Could you check a few things on this model? Use its own coordinates, in mm. Coordinates: 2 decimals unless noted, no trailing zeros. One line per item, written item: value.
Autodesk Inventor part; units mm, degrees
ref_plane "YZ Plane" through (0, 0, 0) normal (1, 0, 0) x (0, 1, 0)
ref_plane "XZ Plane" through (0, 0, 0) normal (0, 1, 0) x (-1, 0, 0)
ref_plane "XY Plane" through (0, 0, 0) normal (0, 0, 1) x (1, 0, 0)
sketch "Sketch1" plane through (0, 0, 0) normal (0, 1, 0) x (-1, 0, 0)
  line L0 (-0.4496, -84) -> (-0.4496, 0)
  line L1 (-120.7289, 0) -> (-120.7289, -84)
  circle A0 centre (-60.5893, -17) radius 7.5
  circle A1 centre (-25.6593, -25) radius 6.5
  circle A2 centre (-95.5193, -25) radius 6.5
  circle A3 centre (-18.1343, -17.5) radius 1.05
  circle A4 centre (-18.1343, -37.5) radius 1.05
  circle A5 centre (-18.1343, -52.6) radius 1.05
  circle A6 centre (-33.1843, -52.6) radius 1.05
  circle A7 centre (-33.1843, -37.5) radius 1.05
  circle A8 centre (-33.1843, -17.5) radius 1.05
  circle A9 centre (-87.9943, -17.5) radius 1.05
  circle A10 centre (-87.9943, -37.5) radius 1.05
  circle A11 centre (-87.9943, -52.6) radius 1.05
  circle A12 centre (-103.0443, -52.6) radius 1.05
  circle A13 centre (-103.0443, -37.5) radius 1.05
  circle A14 centre (-103.0443, -17.5) radius 1.05
  circle A15 centre (-215.8686, -26) radius 1.05
  circle A16 centre (94.69, -26) radius 1.05
  circle A17 centre (-215.8686, -9.86) radius 1.05
  circle A18 centre (94.69, -9.86) radius 1.05
  circle A19 centre (-207.8686, -17.93) radius 6.4
  circle A20 centre (86.69, -17.93) radius 6.4
  circle A21 centre (-188.4636, -49.095) radius 1.55
  circle A22 centre (67.285, -49.095) radius 1.55
  circle A23 centre (-137.4636, -73.095) radius 1.55
  circle A24 centre (16.285, -73.095) radius 1.55
  circle A25 centre (-162.4636, -73.095) radius 1.55
  circle A26 centre (41.285, -73.095) radius 1.55
  circle A27 centre (-139.3686, -40.905) radius 1.55
  circle A28 centre (18.19, -40.905) radius 1.55
  circle A29 centre (-169.3686, -40.905) radius 1.55
  circle A30 centre (48.19, -40.905) radius 1.55
  circle A31 centre (-139.3686, -10.405) radius 1.55
  circle A32 centre (18.19, -10.405) radius 1.55
  circle A33 centre (-169.3686, -10.405) radius 1.55
  circle A34 centre (48.19, -10.405) radius 1.55
  circle A35 centre (-200.9686, -9.93) radius 1.05
  circle A36 centre (-200.9686, -25.93) radius 1.05
  circle A37 centre (-187.7486, -24.93) radius 1.05
  circle A38 centre (-180.4486, -17.93) radius 1.05
  circle A39 centre (-187.7486, -10.93) radius 1.05
  circle A40 centre (79.79, -9.93) radius 1.05
  circle A41 centre (79.79, -25.93) radius 1.05
  circle A42 centre (66.57, -24.93) radius 1.05
  circle A43 centre (59.27, -17.93) radius 1.05
  circle A44 centre (66.57, -10.93) radius 1.05
  arc A45 (-219.3686, -59) -> (-218.3686, -60) centre (-218.3686, -59) ccw
  line L2 (-218.3686, -60) -> (-181.8686, -60)
  arc A46 (-180.8686, -61) -> (-181.8686, -60) centre (-181.8686, -61) ccw
  arc A47 (-180.8686, -83) -> (-179.8686, -84) centre (-179.8686, -83) ccw
  line L3 (-180.8686, -61) -> (-180.8686, -83)
  arc A48 (58.69, -84) -> (59.69, -83) centre (58.69, -83) ccw
  line L4 (59.69, -83) -> (59.69, -61)
  arc A49 (60.69, -60) -> (59.69, -61) centre (60.69, -61) ccw
  line L5 (60.69, -60) -> (97.19, -60)
  arc A50 (97.19, -60) -> (98.19, -59) centre (97.19, -59) ccw
  line L6 (98.19, -1) -> (98.19, -59)
  arc A51 (98.19, -1) -> (97.19, 0) centre (97.19, -1) ccw
  line L7 (-218.3686, 0) -> (97.19, 0)
  arc A52 (-218.3686, 0) -> (-219.3686, -1) centre (-218.3686, -1) ccw
  line L8 (-219.3686, -59) -> (-219.3686, -1)
  line L9 (58.69, -84) -> (-179.8686, -84)
  line L10 (-121.1786, -84) -> (-121.1786, 0)
  line L11 (-120.2793, 0) -> (-120.2793, -84)
  line L12 (-0.8993, -84) -> (-0.8993, 0)
  line L13 (0, 0) -> (0, -84)
  point P0 (0, 0)
extrude "Extrusion1" add sketch "Sketch1" against normal blind 1.5
properties part number "body_main_frame"
Item 1: If I drill on probe 1 along Z at (x, y) = (-48.19, -1.2) (3 decimals); probe 2 along Z at (x, y) = (-18, -0.2); probe 3 along Z at (x, y) = (-66.57, -1.2), over which ranges is the centre line in solid material (lowest first)?
Conclusion:
probe 1: -84 to -42.455, -39.355 to -11.955, -8.855 to 0
probe 2: -84 to -42.44, -39.37 to -11.94, -8.87 to 0
probe 3: -60 to -50.47, -47.72 to -25.98, -23.88 to -11.98, -9.88 to 0
Item 2: I want a section at A-A on y = -0.45. Give the number of separate pieces and of enclosed holes in the cut face, then the cut area to 3 significant figures.
Conclusion:
separate pieces: 1
enclosed holes: 45
area: 23,900 mm²
Item 3: I'm going to push a flat-ended pin straight in: pin 1 Ø11.5 at (x, z) = (-86.69, -17.93) entering from +Y. Where does the tip first touch, or does it pass through?
Conclusion:
pin 1: through
